Build history of the part. All positions in model axes, mm. Face numbers are marked on the shaded views. A direction names the side the tool comes from. Round coordinates to 2 decimals unless told otherwise and drop trailing zeros. Loops run counter-clockwise (first coordinate to the right, second up) from the corner with the lowest first, then second, coordinate; pieces in that order, holes last. Notation, with made-up numbers: (62, -14) - (111, -14) arc R8 ccw to (111, -5) - close; hole circle Ø1 at (-10.75, 80.25). An arc over 180 degrees is marked (long way). Use a Markdown table: item, result.
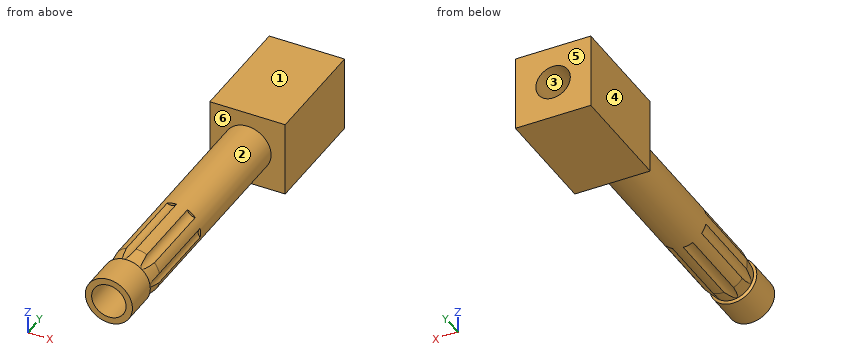
from build123d import *

# Parameters (mm, degrees)
F0_W     = 25.4
F0_H     = 25.4
F0_R     = 7.9375
F0_R_2   = 5.8024107256
F1_DEPTH = 38.1
F2_DEPTH = 127
F6_START = -12.192
F5_R     = 2.4554456834
F6_DEPTH = 31.496


with BuildPart() as f1:
    # F0 (on Front) → F1 (new body)
    with BuildSketch(Plane.XZ):
        Rectangle(F0_W, F0_H)
        Circle(F0_R, mode=Mode.SUBTRACT)
        Circle(F0_R)
        Circle(F0_R_2, mode=Mode.SUBTRACT)
    extrude(amount=F1_DEPTH)

    # F0 (on Front) → F2 (join)
    with BuildSketch(Plane.XZ):
        Circle(F0_R)
        Circle(F0_R_2, mode=Mode.SUBTRACT)
    extrude(amount=F2_DEPTH)

    # F3 (on Top) → F4 (revolve, cut)
    with BuildSketch(Plane.XY):
        Polygon((-8.0296611413, -108.8151410222), (-8.0938637257, -115.6206354499), (-7.0666195825, -115.1070147753), align=None)
    revolve(axis=Axis((0, 0, 0), (0, -1, 0)), mode=Mode.SUBTRACT)

    # F5 (on face) → F6 (cut)
    with BuildSketch(Plane.XZ.offset(127).offset(F6_START)):
        with Locations((9.5767229945, -0.0002272034)):
            Circle(F5_R)
        with Locations((5.9707205281, 7.487714074)):
            Circle(F5_R)
        with Locations((-2.1318934647, 9.3370828434)):
            Circle(F5_R)
        with Locations((-8.6296853842, 4.1552667011)):
            Circle(F5_R)
        with Locations((-8.6296853842, -4.155721108)):
            Circle(F5_R)
        with Locations((-2.1318934647, -9.3375372503)):
            Circle(F5_R)
        with Locations((5.9707205281, -7.4881684809)):
            Circle(F5_R)
    extrude(amount=-F6_DEPTH, mode=Mode.SUBTRACT)


solid = f1.part
Q1. Cut at B-B, the plane z = 0. List the corners of the cut face in (x, y).
Results found:
| item | result |
|---|---|
| outline | (-12.7, -38.1) - (-7.94, -38.1) - (-7.94, -109.42) - (-7.07, -115.11) - (-7.94, -115.54) - (-7.94, -127) - (-5.8, -127) - (-5.8, 0) - (-12.7, 0) - close; (5.8, -127) - (7.94, -127) - (7.94, -115.54) - (7.07, -115.11) - (7.12, -114.75) - (7.12, -83.31) - (7.94, -83.31) - (7.94, -38.1) - (12.7, -38.1) - (12.7, 0) - (5.8, 0) - close |
Q2. Cut at C-C, the plane x = 10.5. List the corners of the cut face in (y, z), plus the area to 3 significant figures.
Results found:
| item | result |
|---|---|
| outline | (-38.1, -12.7) - (0, -12.7) - (0, 12.7) - (-38.1, 12.7) - close |
| area | 968 mm2 |
Q3. Cut at D-D, the plane y = -96.5. List the corners of the cut face in (x, z) (1 decimal).
Results found:
| item | result |
|---|---|
| outline | (-7.7, -1.9) arc R2.5 cw to (-6.3, -4.9) arc R7.9 ccw to (-3.3, -7.2) arc R2.5 cw to (-0.1, -7.9) arc R7.9 ccw to (3.5, -7.1) arc R2.5 cw to (6.1, -5) arc R7.9 ccw to (7.8, -1.7) arc R2.5 cw to (7.8, 1.7) arc R7.9 ccw to (6.1, 5) arc R2.5 cw to (3.5, 7.1) arc R7.9 ccw to (-0.1, 7.9) arc R2.5 cw to (-3.3, 7.2) arc R7.9 ccw to (-6.3, 4.9) arc R2.5 cw to (-7.7, 1.9) arc R7.9 ccw to start; hole circle Ø11.6 at (0, 0) |
Q4. Drop flat-ended pins along their axis: pin 1 (12.5 mm diameter, centred on x = -2, z = -2, fed in from -Y); pin 2 (1.5 mm diameter, centred on y = -40.5, z = -9, fed in from +X); pin 3 (5 mm diameter, centred on y = -93, z = 7, fed in from -X); pin 4 (1.5 mm diameter, centred on y = -67, z = 2.5, fed in from +X). Give the stop position or say it passes through.
Results found:
| item | result |
|---|---|
| pin 1 | stops at y = -127 |
| pin 2 | passes through |
| pin 3 | stops at x = -6.28 |
| pin 4 | stops at x = 7.74 |
Q5. Cut at A-A, the plane y = -28. List the corners of the cut face in (x, z).
Results found:
| item | result |
|---|---|
| outline | (-12.7, -12.7) - (12.7, -12.7) - (12.7, 12.7) - (-12.7, 12.7) - close; hole circle Ø11.6 at (0, 0) |
Q6. Which spindle directions (+Z, -Z, +X, -X, +Y, -Y) get a long thin tool onto all of the face, cutting with end or side? Do the marked faces 5 and 6. Say none if no direction does.
Results found:
| item | result |
|---|---|
| face 5 | +Z, -Z, +X, -X, +Y |
| face 6 | -Y |
Q7. Probe line 1 (Z direction, x = 0, y = -37.5); line 2 (Z direction, x = 0, y = -41.5); line 3 (X direction, y = -37, z = -2). List the from-to ranges inside material, lowest first.
Results found:
| item | result |
|---|---|
| line 1 | z = -12.7 to -5.8, 5.8 to 12.7 |
| line 2 | z = -7.94 to -5.8, 5.8 to 7.94 |
| line 3 | x = -12.7 to -5.45, 5.45 to 12.7 |
Q8. Pull direction Z, two halves, no side cores. Call the marked faces 1, 2, 3 and 4: pulls with the +Z half, pulls with the -Z half, needs draft (parallel to the pull), parting line crosses it, or undercut.
Results found:
| item | result |
|---|---|
| face 1 | pulls with the +Z half |
| face 2 | parting line crosses it |
| face 3 | undercut |
| face 4 | needs draft |
